Part model, mm, in its own coordinate system. A direction names the side the tool comes from. Round coordinates to 2 decimals unless told otherwise and drop trailing zeros. Write each loop counter-clockwise with the first axis right and the second up, starting at its lowest first coordinate (ties: lowest second). Pieces come first, ordered by that corner, then holes.
from build123d import *

# Parameters (mm, degrees)
SKETCH1_R           = 77.5
SKETCH1_R_2         = 70
BOSS_EXTRUDE1_DEPTH = 8
SKETCH2_R           = 1.5
CUT_EXTRUDE1_DEPTH  = 6


with BuildPart() as part:
    # Sketch1 → Boss-Extrude1 (new body)
    with BuildSketch(Plane.XY):
        Polygon((-148.270283039, 111.64556962), (147.729716961, 111.64556962), (147.729716961, 81.64556962), (159.729716961, 81.64556962), (159.729716961, -60.35443038), (-160.270283039, -60.35443038), (-160.270283039, 81.64556962), (-148.270283039, 81.64556962), align=None)
        with Locations((-78.270283039, 25.64556962)):
            Circle(SKETCH1_R, mode=Mode.SUBTRACT)
        with Locations((77.729716961, 25.64556962)):
            Circle(SKETCH1_R_2, mode=Mode.SUBTRACT)
    extrude(amount=BOSS_EXTRUDE1_DEPTH)

    # Sketch2 → Cut-Extrude1 (cut)
    with BuildSketch(Plane.XY):
        with Locations((-0.270283039, 96.64556962)):
            Circle(SKETCH2_R)
        with Locations((144.729716961, -45.35443038)):
            Circle(SKETCH2_R)
        with Locations((-145.270283039, -45.35443038)):
            Circle(SKETCH2_R)
    extrude(amount=CUT_EXTRUDE1_DEPTH, mode=Mode.SUBTRACT)


solid = part.part
Q1. Wall check: line 1 (X direction, y = 40.5, z = 7.5); line 2 (X direction, y = 10, z = 6.5); line 3 (Y direction, x = -133.5, z = 5.75). Give the ranges that are in metal, low to high.
Q2. Two-plate mould, pull along Y, no slides. Class faces 4 (the flat face through (2, -60.354, 4)), 5 (the cylindrical face through (115.36, 84.67, 3.94)), 6 (the flat face through (-2, 111.646, 4)), 7 (the flat face through (-160.27, 10, 4)): released by +Y, released by -Y, zero draft, split by the parting line, or undercut.
Q3. Saw through at D-D, the plane y = -16.5. Write the cut outline in (x, z).
Q4. Tool access for faces 1 (the cylindrical face through (-139.772, -21.512, 3.944)), 2 (the flat face through (147.73, 97, 4)), 3 (the flat face through (-154, 81.646, 4)): list every direction of +Z, -Z, +X, -X, +Y, -Y with a clear straight run to the whole face (end or side of a thin tool).
Q5. Drop flat-ended pins along their axis: P1, Ø4, axis at x = 153, z = 4, coming from the +Y side; P2, Ø0.9, axis at x = -144.5, y = -46, coming from the -Z side. Give the stop position or say it passes through.
Q6. Saw through at B-B, the plane x = 75. Write the cut outline in (y, z).
Q7. Saw through at A-A, the plane y = 31.5. Write the cut outline in (x, z).
Q8. Saw through at C-C, the plane z = 3.25. Write the cut outline in (x, y).
Computed:
1. line 1: x = -160.27 to -154.33, -2.21 to 9.32, 146.14 to 159.73
1. line 2: x = -160.27 to -154.17, -2.37 to 9.5, 145.96 to 159.73
1. line 3: y = -60.35 to -28.72, 80.01 to 111.65
2. face 4: released by -Y
2. face 5: undercut
2. face 6: released by +Y
2. face 7: zero draft
3. outline: (-160.27, 0) - (-143.31, 0) - (-143.31, 8) - (-160.27, 8) - close; (-13.23, 0) - (21.84, 0) - (21.84, 8) - (-13.23, 8) - close; (133.62, 0) - (159.73, 0) - (159.73, 8) - (133.62, 8) - close
4. face 1: +Z, -Z
4. face 2: +Z, -Z, +X, +Y
4. face 3: +Z, -Z, -X, +Y
5. P1: stops at y = 81.65
5. P2: stops at z = 6
6. outline: (-60.35, 0) - (-44.3, 0) - (-44.3, 8) - (-60.35, 8) - close; (95.59, 0) - (111.65, 0) - (111.65, 8) - (95.59, 8) - close
7. outline: (-160.27, 0) - (-155.55, 0) - (-155.55, 8) - (-160.27, 8) - close; (-0.99, 0) - (7.97, 0) - (7.97, 8) - (-0.99, 8) - close; (147.48, 0) - (159.73, 0) - (159.73, 8) - (147.48, 8) - close
8. outline: (-160.27, -60.35) - (159.73, -60.35) - (159.73, 81.65) - (147.73, 81.65) - (147.73, 111.65) - (-148.27, 111.65) - (-148.27, 81.65) - (-160.27, 81.65) - close; hole circle Ø155 at (-78.27, 25.65); hole circle Ø3 at (-145.27, -45.35); hole circle Ø3 at (-0.27, 96.65); hole circle Ø140 at (77.73, 25.65); hole circle Ø3 at (144.73, -45.35)
